```python
from build123d import *

# Parameters (mm, degrees)
F0_R     = 55.435679
F0_R_2   = 40.463585
F1_DEPTH = 25.4
F2_W     = 85.478314
F2_H     = 14.102482
F3_DEPTH = 25.4
F4_W     = 16.404928
F4_H     = 86.62954
F5_DEPTH = 25.4


with BuildPart() as f1:
    # F0 (on Front) → F1 (new body)
    with BuildSketch(Plane.XZ):
        Circle(F0_R)
        Circle(F0_R_2, mode=Mode.SUBTRACT)
    extrude(amount=F1_DEPTH)

    # F2 (on Front) → F3 (join)
    with BuildSketch(Plane.XZ):
        Rectangle(F2_W, F2_H)
    extrude(amount=F3_DEPTH)

    # F4 (on Front) → F5 (join)
    with BuildSketch(Plane.XZ):
        Rectangle(F4_W, F4_H)
    extrude(amount=F5_DEPTH)


solid = f1.part
```
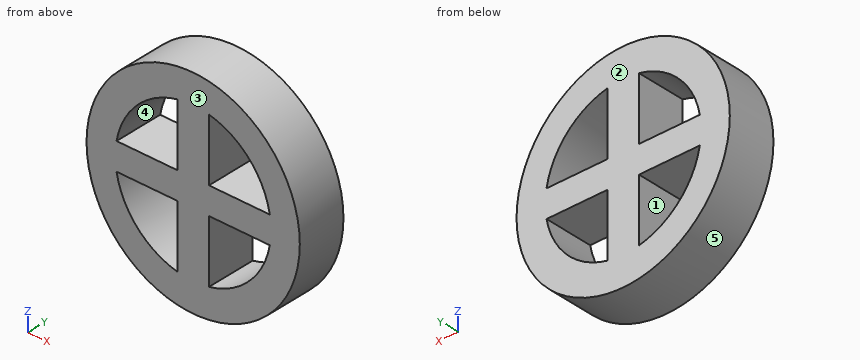
CAD build for the part. Positions are in the model's coordinates, mm. Face numbers are marked on the shaded views. A direction names the side the tool comes from. Round coordinates to 2 decimals unless told otherwise and drop trailing zeros. Order: outer loops, then holes, each group sorted by start corner. A loop starts at its lowest first (then second) coordinate and runs counter-clockwise, first axis right, second up.
Item 1: Pin check, flat tips, straight feed: pin 1 (3 mm diameter, centred on y = -8.5, z = 29.5, fed in from -X); pin 2 (7.5 mm diameter, centred on y = -18.5, z = -20, fed in from -X); pin 3 (12 mm diameter, centred on y = -20, z = -16, fed in from +X); pin 4 (2 mm diameter, centred on x = -40, z = -41.5, fed in from -Y). Stop position of each tip, or through.
Item 2: Saw through at D-D on z = -45.5. Write the cut outline in (x, y), then the cut area to 3 significant figures.
Item 3: Probe line 1 along Z through (x, y) = (14, -18.5); line 2 along Z through (x, y) = (15.5, -9); line 3 along X through (y, z) = (-12, -32.5). List the from-to ranges inside material, lowest first.
Item 4: Tool access for the marked faces 1 and 2: list every direction of +Z, -Z, +X, -X, +Y, -Y with a clear straight run to the whole face (end or side of a thin tool).
Item 5: Saw through at C-C on x = 35.5. Write the cut outline in (y, z), then the cut area to 3 significant figures.
Item 6: Saw through at B-B on z = 38. Write the cut outline in (x, y).
Item 7: Saw through at A-A on y = -5. Write the cut outline in (x, z).
Item 8: Mould opens along X. For the marked faces 3, 4 and 5 say: pulls with the +X half, pulls with the -X half, needs draft (parallel to the pull), parting line crosses it, or undercut.
Reported:
1. pin 1: stops at x = -47.84
1. pin 2: stops at x = -53
1. pin 3: stops at x = 54.53
1. pin 4: passes through
2. outline: (-31.67, -25.4) - (31.67, -25.4) - (31.67, 0) - (-31.67, 0) - close
2. area: 1,610 mm2
3. line 1: z = -53.64 to -37.96, -7.05 to 7.05, 37.96 to 53.64
3. line 2: z = -53.22 to -37.38, -7.05 to 7.05, 37.38 to 53.22
3. line 3: x = -44.91 to -24.11, -8.2 to 8.2, 24.11 to 44.91
4. face 1: +Y, -Y
4. face 2: +Z, -Z, +X, -X, +Y
5. outline: (-25.4, -42.58) - (0, -42.58) - (0, -19.42) - (-25.4, -19.42) - close; (-25.4, -7.05) - (0, -7.05) - (0, 7.05) - (-25.4, 7.05) - close; (-25.4, 19.42) - (0, 19.42) - (0, 42.58) - (-25.4, 42.58) - close
5. area: 1,530 mm2
6. outline: (-40.36, -25.4) - (-13.9, -25.4) - (-13.9, 0) - (-40.36, 0) - close; (-8.2, -25.4) - (8.2, -25.4) - (8.2, 0) - (-8.2, 0) - close; (13.9, -25.4) - (40.36, -25.4) - (40.36, 0) - (13.9, 0) - close
7. outline: circle Ø110.87 at (0, 0); hole (-39.84, -7.05) arc R40.46 ccw to (-8.2, -39.62) - (-8.2, -7.05) - close; hole (-39.84, 7.05) - (-8.2, 7.05) - (-8.2, 39.62) arc R40.46 ccw to start; hole (8.2, -39.62) arc R40.46 ccw to (39.84, -7.05) - (8.2, -7.05) - close; hole (8.2, 7.05) - (39.84, 7.05) arc R40.46 ccw to (8.2, 39.62) - close
8. face 3: needs draft
8. face 4: undercut
8. face 5: parting line crosses it
